Source: three-view drawing plus pictorial views. Frame: mm from the lowest corner of the part. A direction names the side the tool comes from. Give positions to 0.01 mm unless a question says otherwise; leave off trailing zeros. Loops run counter-clockwise (first coordinate to the right, second up) from the corner with the lowest first, then second, coordinate; pieces in that order, holes last. Notation, with made-up numbers: M 38,66.5 L 70,66.5 A14 cw 70,74.5 Z; hole C -36,-36 d10. An arc over 180 degrees is marked long. One line per item, written item: value. Start each with the question number.
(1) Section C-C on z = 16.75. Output: boundary loops of the cut face in (x, y), plus the area to 3 significant figures.
(2) Pin query (flat end, axial travel): P1, Ø4, axis at x = 21.5, y = 42, coming from the -Z side; P2, Ø3, axis at x = 30, y = 41.3, coming from the +Z side. Return the tip coordinate at first contact, or that it passes through.
(3) Section D-D on x = 20. Output: boundary loops of the cut face in (y, z).
(4) Ray query, line 1 along X through (y, z) = (15.3, 16); line 2 along Y through (x, z) = (30, 18.75); line 3 along X through (y, z) = (26.5, 7). Return the intervals inside material, ascending. Write a range as from..to.
(5) Access query for the marked faces 5 and 6. Directions: +Z, -Z, +X, -X, +Y, -Y. A direction counts if a zero-diameter tool reaches every point of the face in a straight line with its end or side. Return the directions, or none.
(6) Section B-B on y = 6.5. Output: boundary loops of the cut face in (x, z), plus the area to 3 significant figures.
(7) Section A-A on z = 8. Output: boundary loops of the cut face in (x, y).
(8) Pull-direction query (X, two-part tool) for the marked faces 1, 2, 3 and 4; classes: released by +X, released by -X, zero draft, split by the parting line, or undercut.
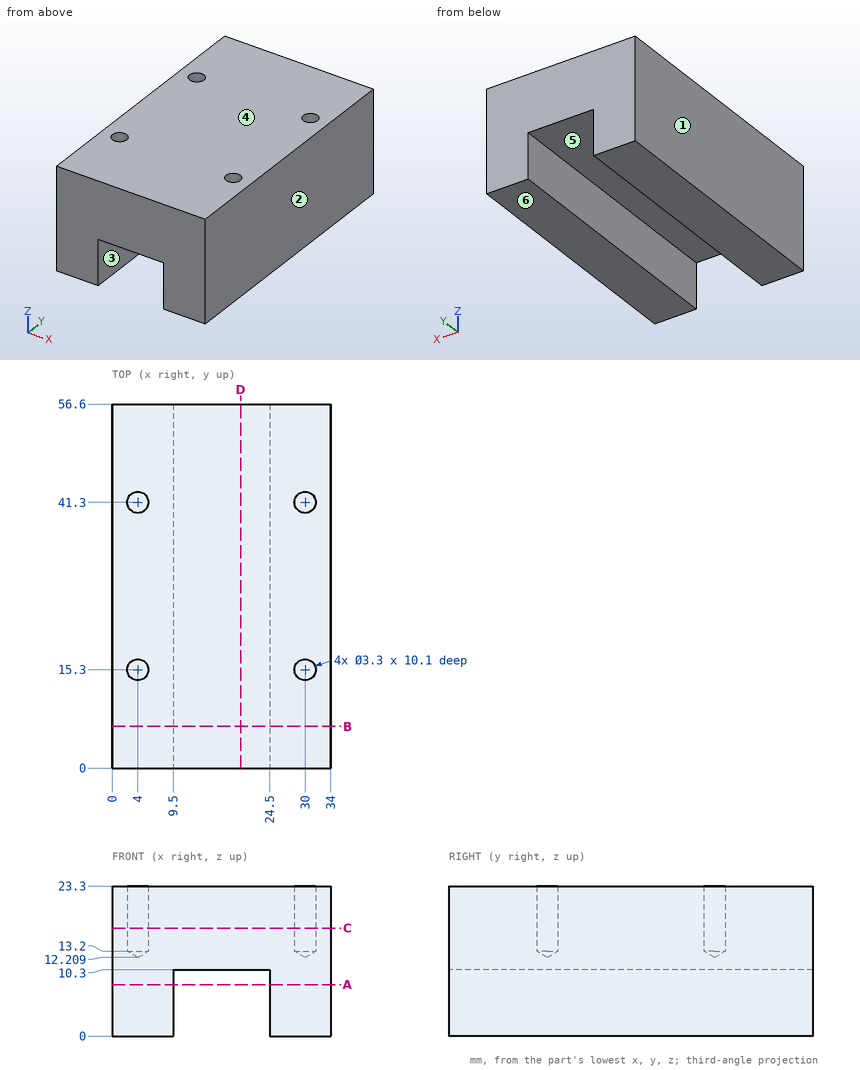
Output values:
1. outline: M 0,0 L 34,0 L 34,56.6 L 0,56.6 Z; hole C 4,15.3 d3.3; hole C 4,41.3 d3.3; hole C 30,15.3 d3.3; hole C 30,41.3 d3.3
1. area: 1,890 mm²
2. P1: stops at z = 10.3
2. P2: stops at z = 13.11
3. outline: M 0,10.3 L 56.6,10.3 L 56.6,23.3 L 0,23.3 Z
4. line 1: x = 0..2.35, 5.65..28.35, 31.65..34
4. line 2: y = 0..13.65, 16.95..39.65, 42.95..56.6
4. line 3: x = 0..9.5, 24.5..34
5. face 5: -Z, +Y, -Y
5. face 6: -Z, +X, -X, +Y, -Y
6. outline: M 0,0 L 9.5,0 L 9.5,10.3 L 24.5,10.3 L 24.5,0 L 34,0 L 34,23.3 L 0,23.3 Z
6. area: 638 mm²
7. outline: M 0,0 L 9.5,0 L 9.5,56.6 L 0,56.6 Z; M 24.5,0 L 34,0 L 34,56.6 L 24.5,56.6 Z
8. face 1: released by -X
8. face 2: released by +X
8. face 3: undercut
8. face 4: zero draft
